from build123d import *

# Parameters (mm, degrees)
F1_DEPTH = 5
F2_R     = 5.08
F3_R     = 1.27
F4_W     = 6.35
F4_H     = 1.016
F5_DEPTH = 3.048
F6_W     = 6.35
F6_H     = 1.778
F7_DEPTH = 1.524
F8_SIZE  = 0.762


with BuildPart() as f1:
    # F0 (on Top) → F1 (new body)
    with BuildSketch(Plane.XY):
        with BuildLine():
            ThreePointArc((-0.949158, 0), (0.066842, 4.333813), (1.082842, 0))
            Line((1.082842, 0), (1.117634, -4.064))
            Line((1.117634, -4.064), (13.817634, -4.064))
            Line((13.817634, -4.064), (13.817634, 8.636))
            Line((13.817634, 8.636), (-13.649158, 8.636))
            Line((-13.649158, 8.636), (-13.649158, -4.064))
            Line((-13.649158, -4.064), (-0.949158, -4.064))
            Line((-0.949158, -4.064), (-0.949158, 0))
        make_face()
    extrude(amount=F1_DEPTH)

    # F2
    f2_edges = [f1.edges().sort_by_distance(p)[0] for p in [
        (-13.649158, 8.636, 2.5),
        (13.817634, 8.636, 2.5),
        (13.817634, -4.064, 2.5),
        (-13.649158, -4.064, 2.5),
    ]]
    fillet(f2_edges, radius=F2_R)

    # F3
    f3_edges = [f1.edges().sort_by_distance(p)[0] for p in [
        (1.117634, -4.064, 2.5),
        (-0.949158, -4.064, 2.5),
    ]]
    fillet(f3_edges, radius=F3_R)

    # F4 (on face) → F5 (join)
    with BuildSketch(Plane.XY.offset(5)):
        with Locations((-8.188158, 0.254)):
            Rectangle(F4_W, F4_H)
        with Locations((-8.188158, 4.318)):
            Rectangle(F4_W, F4_H)
        with Locations((8.321842, 4.318)):
            Rectangle(F4_W, F4_H)
        with Locations((8.321842, 0.254)):
            Rectangle(F4_W, F4_H)
    extrude(amount=F5_DEPTH)

    # F6 (on face) → F7 (join)
    with BuildSketch(Plane.XY.offset(8.048)):
        with Locations((-8.188158, 4.699)):
            Rectangle(F6_W, F6_H)
        with Locations((-8.188158, -0.127)):
            Rectangle(F6_W, F6_H)
        with Locations((8.321842, 4.699)):
            Rectangle(F6_W, F6_H)
        with Locations((8.321842, -0.127)):
            Rectangle(F6_W, F6_H)
    extrude(amount=F7_DEPTH)

    # F8
    f8_edges = [f1.edges().sort_by_distance(p)[0] for p in [
        (-8.188158, -1.016, 9.572),
        (-8.188158, 5.588, 9.572),
        (8.321842, 5.588, 9.572),
        (8.321842, -1.016, 9.572),
    ]]
    chamfer(f8_edges, length=F8_SIZE)


solid = f1.part
Part model, mm, in its own coordinate system. A direction names the side the tool comes from. Coordinates: 2 decimals unless noted, no trailing zeros. Order: outer loops, then holes, each group sorted by start corner. A loop starts at its lowest first (then second) coordinate and runs counter-clockwise, first axis right, second up.
(1) Pull direction Y, two halves, no side cores. Call faces 5 (the face through (-8, 4, 9.572)), 6 (the face through (8, -0.254, 7)), 7 (the face through (8, 0.762, 7)), 8 (the face through (0, 8.636, 2)): pulls with the +Y half, pulls with the -Y half, needs draft (parallel to the pull), parting line crosses it, or undercut.
Check sheet entries:
face 5: needs draft
face 6: pulls with the -Y half
face 7: undercut
face 8: pulls with the +Y half
(2) Slice it at C-C, the plane y = 5.25. Write the cut outline in (x, z), and give its area (3 significant figures).
Check sheet entries:
outline: (-13.36, 0) - (13.53, 0) - (13.53, 5) - (-13.36, 5) - close; (-11.36, 8.05) - (-5.01, 8.05) - (-5.01, 9.15) - (-11.36, 9.15) - close; (5.15, 8.05) - (11.5, 8.05) - (11.5, 9.15) - (5.15, 9.15) - close
area: 148 mm2
(3) Slice it at B-B, the plane x = -5.75. Write the cut outline in (y, z), and give its area (3 significant figures).
Check sheet entries:
outline: (-4.06, 0) - (8.64, 0) - (8.64, 5) - (4.83, 5) - (4.83, 8.05) - (5.59, 8.05) - (5.59, 8.81) - (4.83, 9.57) - (3.81, 9.57) - (3.81, 5) - (0.76, 5) - (0.76, 9.57) - (-0.25, 9.57) - (-1.02, 8.81) - (-1.02, 8.05) - (-0.25, 8.05) - (-0.25, 5) - (-4.06, 5) - close
area: 74.5 mm2
(4) Tool access for faces 1 (the face through (-11.363, 0, 8)), 2 (the face through (-5.013, 0, 8)), 3 (the face through (1.493, -3.706, 2.535)), 4 (the face through (-8, 0.762, 7)): list every direction of +Z, -Z, +X, -X, +Y, -Y with a clear straight run to the whole face (end or side of a thin tool).
Check sheet entries:
face 1: +Z, -X, +Y, -Y
face 2: +Z, +Y, -Y
face 3: +Z, -Z, -Y
face 4: +Z, +X, -X
(5) Slice it at A-A, the plane z = 7. Write the cut outline in (x, y), and give its area (3 significant figures).
Check sheet entries:
outline: (-11.36, -0.25) - (-5.01, -0.25) - (-5.01, 0.76) - (-11.36, 0.76) - close; (-11.36, 3.81) - (-5.01, 3.81) - (-5.01, 4.83) - (-11.36, 4.83) - close; (5.15, -0.25) - (11.5, -0.25) - (11.5, 0.76) - (5.15, 0.76) - close; (5.15, 3.81) - (11.5, 3.81) - (11.5, 4.83) - (5.15, 4.83) - close
area: 25.8 mm2
(6) Probe L1, parallel to Y at x = 9.5, z = 8; L2, parallel to Y at x = 6, z = 8.25; L3, parallel to Z at x = -6.5, y = -3.5. List the from-to ranges inside material, lowest first.
Check sheet entries:
L1: y = -0.25 to 0.76, 3.81 to 4.83
L2: y = -1.02 to 0.76, 3.81 to 5.59
L3: z = 0 to 5
(7) Pin check, flat tips, straight feed: pin 1 Ø3 at (x, y) = (6.5, -2) entering from +Z; pin 2 Ø1 at (x, y) = (0.5, 1) entering from +Z; pin 3 Ø1.4 at (y, z) = (4.5, 6) entering from -X; pin 4 Ø1 at (y, z) = (7, 1.5) entering from +X. Stop position of each tip, or through.
Check sheet entries:
pin 1: stops at z = 9.33
pin 2: passes through
pin 3: stops at x = -11.36
pin 4: stops at x = 12.88
(8) Slice it at D-D, the plane y = 3. Write the cut outline in (x, z).
Check sheet entries:
outline: (-13.65, 0) - (-2.01, 0) - (-2.01, 5) - (-13.65, 5) - close; (2.15, 0) - (13.82, 0) - (13.82, 5) - (2.15, 5) - close
